Part model, mm, in its own coordinate system. A direction names the side the tool comes from. Coordinates: 2 decimals unless noted, no trailing zeros. Loops run counter-clockwise (first coordinate to the right, second up) from the corner with the lowest first, then second, coordinate; pieces in that order, holes last.
```python
from build123d import *

# Parameters (mm, degrees)
SKETCH1_R                                   = 79
SKETCH1_R_2                                 = 6
BOSS_EXTRUDE1_DEPTH                         = 27
CBORE_FOR_0_BINDING_HEAD_MACHINE_SC_2_COUNT = 2
CBORE_FOR_0_BINDING_HEAD_MACHINE_SC_2_PITCH = 64
CBORE_FOR_0_BINDING_HEAD_MACHINE_SC_3_COUNT = 2
CBORE_FOR_0_BINDING_HEAD_MACHINE_SC_3_PITCH = 110.851251684
CBORE_FOR_0_BINDING_HEAD_MACHINE_SC_4_COUNT = 2
CBORE_FOR_0_BINDING_HEAD_MACHINE_SC_4_PITCH = 128
CBORE_FOR_0_BINDING_HEAD_MACHINE_SC_5_COUNT = 2
CBORE_FOR_0_BINDING_HEAD_MACHINE_SC_5_PITCH = 110.851251684
CBORE_FOR_0_BINDING_HEAD_MACHINE_SC_6_COUNT = 2
CBORE_FOR_0_BINDING_HEAD_MACHINE_SC_6_PITCH = 64
CBORE_FOR_0_BINDING_HEAD_MACHINE_SC_7_COUNT = 2
CBORE_FOR_0_BINDING_HEAD_MACHINE_SC_7_PITCH = 64
F_97_0_0059_DIAMETER_HOLE1_D                = 13.99999994
F_97_0_0059_DIAMETER_HOLE1_DEPTH            = 17
F_97_0_0059_DIAMETER_HOLE1_CSINK_D          = 20.8026
F_97_0_0059_DIAMETER_HOLE1_CSINK_ANGLE      = 100
F_97_0_0059_DIAMETER_HOLE1_TIP              = 4.206024315


with BuildPart() as part:
    # Sketch1 → Boss-Extrude1 (new body)
    with BuildSketch(Plane(origin=(0, 0, 0), x_dir=(1, 0, 0), z_dir=(0, 1, 0))):
        Circle(SKETCH1_R)
        Circle(SKETCH1_R_2, mode=Mode.SUBTRACT)
    extrude(amount=BOSS_EXTRUDE1_DEPTH)

    # Sketch5 → CBORE for #0 Binding Head Machine Screw1 (revolve, cut)
    with BuildSketch(Plane(origin=(31.838574382, 27, -55.51851206), x_dir=(0, 0, 1), z_dir=(1, 0, 0))):
        Polygon((0, 0), (0, 27), (6.249999946, 27), (6.249999946, 12.499999892), (9.625000054, 12.499999892), (9.625000054, 0.651392998), (10.4013, 0), align=None)
    cbore_for_0_binding_head_machine_screw1 = revolve(axis=Axis((31.838574382, 33.35, -55.51851206), (0, -1, 0)), mode=Mode.SUBTRACT)

    # CBORE for _0 Binding Head Machine Sc 2: CBORE for #0 Binding Head Machine Screw1 ×2
    with Locations(*[Vector(0.502518041, 0, 0.864566723) * (i * CBORE_FOR_0_BINDING_HEAD_MACHINE_SC_2_PITCH) for i in range(1, CBORE_FOR_0_BINDING_HEAD_MACHINE_SC_2_COUNT)]):
        add(cbore_for_0_binding_head_machine_screw1, mode=Mode.SUBTRACT)

    # CBORE for _0 Binding Head Machine Sc 3: CBORE for #0 Binding Head Machine Screw1 ×2
    with Locations(*[Vector(0.002910028, 0, 0.999995766) * (i * CBORE_FOR_0_BINDING_HEAD_MACHINE_SC_3_PITCH) for i in range(1, CBORE_FOR_0_BINDING_HEAD_MACHINE_SC_3_COUNT)]):
        add(cbore_for_0_binding_head_machine_screw1, mode=Mode.SUBTRACT)

    # CBORE for _0 Binding Head Machine Sc 4: CBORE for #0 Binding Head Machine Screw1 ×2
    with Locations(*[Vector(-0.497477725, 0, 0.867476751) * (i * CBORE_FOR_0_BINDING_HEAD_MACHINE_SC_4_PITCH) for i in range(1, CBORE_FOR_0_BINDING_HEAD_MACHINE_SC_4_COUNT)]):
        add(cbore_for_0_binding_head_machine_screw1, mode=Mode.SUBTRACT)

    # CBORE for _0 Binding Head Machine Sc 5: CBORE for #0 Binding Head Machine Screw1 ×2
    with Locations(*[Vector(-0.864566723, 0, 0.502518041) * (i * CBORE_FOR_0_BINDING_HEAD_MACHINE_SC_5_PITCH) for i in range(1, CBORE_FOR_0_BINDING_HEAD_MACHINE_SC_5_COUNT)]):
        add(cbore_for_0_binding_head_machine_screw1, mode=Mode.SUBTRACT)

    # CBORE for _0 Binding Head Machine Sc 6: CBORE for #0 Binding Head Machine Screw1 ×2
    with Locations(*[Vector(-0.999995766, 0, 0.002910028) * (i * CBORE_FOR_0_BINDING_HEAD_MACHINE_SC_6_PITCH) for i in range(1, CBORE_FOR_0_BINDING_HEAD_MACHINE_SC_6_COUNT)]):
        add(cbore_for_0_binding_head_machine_screw1, mode=Mode.SUBTRACT)

    # CBORE for _0 Binding Head Machine Sc 7: CBORE for #0 Binding Head Machine Screw1 ×2
    with Locations(*[Vector(-0.497477725, 0, 0.867476751) * (i * CBORE_FOR_0_BINDING_HEAD_MACHINE_SC_7_PITCH) for i in range(1, CBORE_FOR_0_BINDING_HEAD_MACHINE_SC_7_COUNT)]):
        add(cbore_for_0_binding_head_machine_screw1, mode=Mode.SUBTRACT)

    # #97 (0.0059) Diameter Hole1
    with Locations(Plane(origin=(0, 27, 0), x_dir=(1, 0, 0), z_dir=(0, 1, 0))):
        with Locations((34, 0)):
            CounterSinkHole(F_97_0_0059_DIAMETER_HOLE1_D / 2, F_97_0_0059_DIAMETER_HOLE1_CSINK_D / 2, depth=F_97_0_0059_DIAMETER_HOLE1_DEPTH, counter_sink_angle=F_97_0_0059_DIAMETER_HOLE1_CSINK_ANGLE)
            with Locations((0, 0, -(F_97_0_0059_DIAMETER_HOLE1_DEPTH + F_97_0_0059_DIAMETER_HOLE1_TIP / 2))):  # 118° drill point
                Cone(0, F_97_0_0059_DIAMETER_HOLE1_D / 2, F_97_0_0059_DIAMETER_HOLE1_TIP, mode=Mode.SUBTRACT)


solid = part.part
```
Q1. Mould opens along Z. For faces 3 (the flat face through (-1, 0, 16)), 4 (the flat face through (32, 14.5, -62)) say: released by +Z, released by -Z, zero draft, split by the parting line, or undercut.
Q2. Probe line 1 (X direction, y = 18.25, z = -0.5); line 2 (X direction, y = 20.75, z = 61); line 3 (X direction, y = 24.75, z = -56.5). List the from-to ranges inside material, lowest first.
Q3. Tool access for faces 1 (the cylindrical face through (-41.382, 20.507, 54.266)), 2 (the cylindrical face through (-33.72, 7.35, 61.48)): list every direction of +Z, -Z, +X, -X, +Y, -Y with a clear straight run to the whole face (end or side of a thin tool).
Q4. Saw through at B-B (z = -3.5). Count the separate pieces of the cut face and the enclosed holes in it, plus the area to 3 significant figures.
Q5. Drop flat-ended pins along their axis: P1, Ø6, axis at x = -59, z = 3.5, coming from the +Y side; P2, Ø25, axis at x = -64, z = 0.19, coming from the +Y side; P3, Ø10, axis at y = 12, z = 55.5, coming from the +X side; P4, Ø2, axis at x = 8.5, y = 11.5, coming from the -Z side. Give the stop position or say it passes through.
Q6. Saw through at D-D (x = 49.5). List the corners of the cut face in (y, z).
Q7. Saw through at A-A (x = 0). List the corners of the cut face in (y, z) (3 decimals).
Checked values:
1. face 3: zero draft
1. face 4: undercut
2. line 1: x = -79 to -73.6, -54.4 to -9.61, 9.61 to 27.02, 40.98 to 54.38, 73.62 to 79
2. line 2: x = -50.2 to -39.75, -23.93 to 24.38, 39.94 to 50.2
2. line 3: x = -55.22 to -41.72, -22.61 to 22.26, 41.41 to 55.22
3. face 1: +Y
3. face 2: +Y, -Y
4. separate pieces: 4
4. enclosed holes: 0
4. area: 2,900 mm2
5. P1: stops at y = 14.5
5. P2: stops at y = 27
5. P3: stops at x = 60.75
5. P4: stops at z = -78.64
6. outline: (0, -61.57) - (27, -61.57) - (27, 61.57) - (0, 61.57) - close
7. outline: (0, -79) - (27, -79) - (27, -10.401) - (26.349, -9.625) - (14.5, -9.625) - (14.5, -6.25) - (0, -6.25) - close; (0, 6.25) - (14.5, 6.25) - (14.5, 9.625) - (26.349, 9.625) - (27, 10.401) - (27, 79) - (0, 79) - close
